Source: CAD feature listing. Evaluate the final solid. Frame: model axes, mm. Coordinates: 2 decimals unless noted, no trailing zeros. Loops run counter-clockwise (first coordinate to the right, second up) from the corner with the lowest first, then second, coordinate; pieces in that order, holes last. Notation, with made-up numbers: (48, 14.25) - (66, 14.25) arc R17 cw to (66, 30.25) - close; hole circle Ø11 at (71.25, 0.25). An arc over 180 degrees is marked (long way). Use CSV: the item, a comma, the result in double quotes. Start each with the question number.
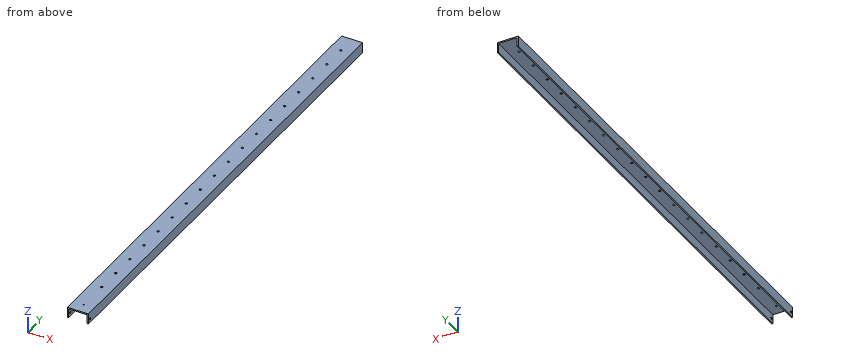
```python
from build123d import *

# Parameters (mm, degrees)
BOSS_EXTRUDE1_DEPTH = 1168.4
IGUS_HOLES_REACH    = 27.4
SKETCH2_R           = 2.667
CUT_EXTRUDE2_REACH  = 5.175
SKETCH3_R           = 1.5875
SKETCH4_R           = 2.667
CUT_EXTRUDE3_DEPTH  = 51.8


with BuildPart() as part:
    # Sketch1 → Boss-Extrude1 (new body)
    with BuildSketch(Plane(origin=(0, 0, 0), x_dir=(1, 0, 0), z_dir=(0, 1, 0))):
        Polygon((3.175, 3.175), (3.175, 25.4), (0, 25.4), (0, 0), (50.8, 0), (50.8, 25.4), (47.625, 25.4), (47.625, 3.175), align=None)
    extrude(amount=BOSS_EXTRUDE1_DEPTH)

    # Sketch2 → Igus_Holes (cut, up to next)
    with BuildSketch(Plane.XY, mode=Mode.PRIVATE) as igus_holes_sk1:
        with Locations((25.4, 101.6)):
            Circle(SKETCH2_R)
    igus_holes_tool1 = extrude(igus_holes_sk1.sketch, amount=-IGUS_HOLES_REACH, mode=Mode.PRIVATE) & part.part
    add(igus_holes_tool1.solids().sort_by_distance((25.4, 101.6, 0))[0], mode=Mode.SUBTRACT)
    # Sketch2 → Igus_Holes (cut, up to next)
    with BuildSketch(Plane.XY, mode=Mode.PRIVATE) as igus_holes_sk2:
        with Locations((25.4, 161.544)):
            Circle(SKETCH2_R)
    igus_holes_tool2 = extrude(igus_holes_sk2.sketch, amount=-IGUS_HOLES_REACH, mode=Mode.PRIVATE) & part.part
    add(igus_holes_tool2.solids().sort_by_distance((25.4, 161.544, 0))[0], mode=Mode.SUBTRACT)
    # Sketch2 → Igus_Holes (cut, up to next)
    with BuildSketch(Plane.XY, mode=Mode.PRIVATE) as igus_holes_sk3:
        with Locations((25.4, 221.488)):
            Circle(SKETCH2_R)
    igus_holes_tool3 = extrude(igus_holes_sk3.sketch, amount=-IGUS_HOLES_REACH, mode=Mode.PRIVATE) & part.part
    add(igus_holes_tool3.solids().sort_by_distance((25.4, 221.488, 0))[0], mode=Mode.SUBTRACT)
    # Sketch2 → Igus_Holes (cut, up to next)
    with BuildSketch(Plane.XY, mode=Mode.PRIVATE) as igus_holes_sk4:
        with Locations((25.4, 281.432)):
            Circle(SKETCH2_R)
    igus_holes_tool4 = extrude(igus_holes_sk4.sketch, amount=-IGUS_HOLES_REACH, mode=Mode.PRIVATE) & part.part
    add(igus_holes_tool4.solids().sort_by_distance((25.4, 281.432, 0))[0], mode=Mode.SUBTRACT)
    # Sketch2 → Igus_Holes (cut, up to next)
    with BuildSketch(Plane.XY, mode=Mode.PRIVATE) as igus_holes_sk5:
        with Locations((25.4, 341.376)):
            Circle(SKETCH2_R)
    igus_holes_tool5 = extrude(igus_holes_sk5.sketch, amount=-IGUS_HOLES_REACH, mode=Mode.PRIVATE) & part.part
    add(igus_holes_tool5.solids().sort_by_distance((25.4, 341.376, 0))[0], mode=Mode.SUBTRACT)
    # Sketch2 → Igus_Holes (cut, up to next)
    with BuildSketch(Plane.XY, mode=Mode.PRIVATE) as igus_holes_sk6:
        with Locations((25.4, 401.32)):
            Circle(SKETCH2_R)
    igus_holes_tool6 = extrude(igus_holes_sk6.sketch, amount=-IGUS_HOLES_REACH, mode=Mode.PRIVATE) & part.part
    add(igus_holes_tool6.solids().sort_by_distance((25.4, 401.32, 0))[0], mode=Mode.SUBTRACT)
    # Sketch2 → Igus_Holes (cut, up to next)
    with BuildSketch(Plane.XY, mode=Mode.PRIVATE) as igus_holes_sk7:
        with Locations((25.4, 461.264)):
            Circle(SKETCH2_R)
    igus_holes_tool7 = extrude(igus_holes_sk7.sketch, amount=-IGUS_HOLES_REACH, mode=Mode.PRIVATE) & part.part
    add(igus_holes_tool7.solids().sort_by_distance((25.4, 461.264, 0))[0], mode=Mode.SUBTRACT)
    # Sketch2 → Igus_Holes (cut, up to next)
    with BuildSketch(Plane.XY, mode=Mode.PRIVATE) as igus_holes_sk8:
        with Locations((25.4, 521.208)):
            Circle(SKETCH2_R)
    igus_holes_tool8 = extrude(igus_holes_sk8.sketch, amount=-IGUS_HOLES_REACH, mode=Mode.PRIVATE) & part.part
    add(igus_holes_tool8.solids().sort_by_distance((25.4, 521.208, 0))[0], mode=Mode.SUBTRACT)
    # Sketch2 → Igus_Holes (cut, up to next)
    with BuildSketch(Plane.XY, mode=Mode.PRIVATE) as igus_holes_sk9:
        with Locations((25.4, 581.152)):
            Circle(SKETCH2_R)
    igus_holes_tool9 = extrude(igus_holes_sk9.sketch, amount=-IGUS_HOLES_REACH, mode=Mode.PRIVATE) & part.part
    add(igus_holes_tool9.solids().sort_by_distance((25.4, 581.152, 0))[0], mode=Mode.SUBTRACT)
    # Sketch2 → Igus_Holes (cut, up to next)
    with BuildSketch(Plane.XY, mode=Mode.PRIVATE) as igus_holes_sk10:
        with Locations((25.4, 641.096)):
            Circle(SKETCH2_R)
    igus_holes_tool10 = extrude(igus_holes_sk10.sketch, amount=-IGUS_HOLES_REACH, mode=Mode.PRIVATE) & part.part
    add(igus_holes_tool10.solids().sort_by_distance((25.4, 641.096, 0))[0], mode=Mode.SUBTRACT)
    # Sketch2 → Igus_Holes (cut, up to next)
    with BuildSketch(Plane.XY, mode=Mode.PRIVATE) as igus_holes_sk11:
        with Locations((25.4, 701.04)):
            Circle(SKETCH2_R)
    igus_holes_tool11 = extrude(igus_holes_sk11.sketch, amount=-IGUS_HOLES_REACH, mode=Mode.PRIVATE) & part.part
    add(igus_holes_tool11.solids().sort_by_distance((25.4, 701.04, 0))[0], mode=Mode.SUBTRACT)
    # Sketch2 → Igus_Holes (cut, up to next)
    with BuildSketch(Plane.XY, mode=Mode.PRIVATE) as igus_holes_sk12:
        with Locations((25.4, 760.984)):
            Circle(SKETCH2_R)
    igus_holes_tool12 = extrude(igus_holes_sk12.sketch, amount=-IGUS_HOLES_REACH, mode=Mode.PRIVATE) & part.part
    add(igus_holes_tool12.solids().sort_by_distance((25.4, 760.984, 0))[0], mode=Mode.SUBTRACT)
    # Sketch2 → Igus_Holes (cut, up to next)
    with BuildSketch(Plane.XY, mode=Mode.PRIVATE) as igus_holes_sk13:
        with Locations((25.4, 820.928)):
            Circle(SKETCH2_R)
    igus_holes_tool13 = extrude(igus_holes_sk13.sketch, amount=-IGUS_HOLES_REACH, mode=Mode.PRIVATE) & part.part
    add(igus_holes_tool13.solids().sort_by_distance((25.4, 820.928, 0))[0], mode=Mode.SUBTRACT)
    # Sketch2 → Igus_Holes (cut, up to next)
    with BuildSketch(Plane.XY, mode=Mode.PRIVATE) as igus_holes_sk14:
        with Locations((25.4, 880.872)):
            Circle(SKETCH2_R)
    igus_holes_tool14 = extrude(igus_holes_sk14.sketch, amount=-IGUS_HOLES_REACH, mode=Mode.PRIVATE) & part.part
    add(igus_holes_tool14.solids().sort_by_distance((25.4, 880.872, 0))[0], mode=Mode.SUBTRACT)
    # Sketch2 → Igus_Holes (cut, up to next)
    with BuildSketch(Plane.XY, mode=Mode.PRIVATE) as igus_holes_sk15:
        with Locations((25.4, 940.816)):
            Circle(SKETCH2_R)
    igus_holes_tool15 = extrude(igus_holes_sk15.sketch, amount=-IGUS_HOLES_REACH, mode=Mode.PRIVATE) & part.part
    add(igus_holes_tool15.solids().sort_by_distance((25.4, 940.816, 0))[0], mode=Mode.SUBTRACT)
    # Sketch2 → Igus_Holes (cut, up to next)
    with BuildSketch(Plane.XY, mode=Mode.PRIVATE) as igus_holes_sk16:
        with Locations((25.4, 1000.76)):
            Circle(SKETCH2_R)
    igus_holes_tool16 = extrude(igus_holes_sk16.sketch, amount=-IGUS_HOLES_REACH, mode=Mode.PRIVATE) & part.part
    add(igus_holes_tool16.solids().sort_by_distance((25.4, 1000.76, 0))[0], mode=Mode.SUBTRACT)
    # Sketch2 → Igus_Holes (cut, up to next)
    with BuildSketch(Plane.XY, mode=Mode.PRIVATE) as igus_holes_sk17:
        with Locations((25.4, 1060.704)):
            Circle(SKETCH2_R)
    igus_holes_tool17 = extrude(igus_holes_sk17.sketch, amount=-IGUS_HOLES_REACH, mode=Mode.PRIVATE) & part.part
    add(igus_holes_tool17.solids().sort_by_distance((25.4, 1060.704, 0))[0], mode=Mode.SUBTRACT)
    # Sketch2 → Igus_Holes (cut, up to next)
    with BuildSketch(Plane.XY, mode=Mode.PRIVATE) as igus_holes_sk18:
        with Locations((25.4, 1120.648)):
            Circle(SKETCH2_R)
    igus_holes_tool18 = extrude(igus_holes_sk18.sketch, amount=-IGUS_HOLES_REACH, mode=Mode.PRIVATE) & part.part
    add(igus_holes_tool18.solids().sort_by_distance((25.4, 1120.648, 0))[0], mode=Mode.SUBTRACT)

    # Sketch3 → Cut-Extrude2 (cut, up to next)
    with BuildSketch(Plane(origin=(0, 0, -3.175), x_dir=(-1, 0, 0), z_dir=(0, 0, -1)), mode=Mode.PRIVATE) as cut_extrude2_sk1:
        with Locations((-25.4, 25.4)):
            Circle(SKETCH3_R)
    cut_extrude2_tool1 = extrude(cut_extrude2_sk1.sketch, amount=-CUT_EXTRUDE2_REACH, mode=Mode.PRIVATE) & part.part
    add(cut_extrude2_tool1.solids().sort_by_distance((25.4, 25.4, -3.175))[0], mode=Mode.SUBTRACT)

    # Sketch4 → Cut-Extrude3 (cut, through all)
    with BuildSketch(Plane.ZY):
        with Locations((-15.875, 6.35)):
            Circle(SKETCH4_R)
    extrude(amount=-CUT_EXTRUDE3_DEPTH, mode=Mode.SUBTRACT)


solid = part.part
```
(1) Pin query (flat end, axial travel): pin 1 Ø7 at (x, y) = (25.4, 341.376) entering from -Z (3 decimals). Return the tip coordinate at first contact, or that it passes through.
(2) Section B-B on y = 131. Output: boundary loops of the cut face in (x, z) (3 decimals), plus the area to 3 significant figures.
(3) Section A-A on z = -8. Output: boundary loops of the cut face in (x, y) (3 decimals), plus the area to 3 significant figures.
(4) Ray query, line 1 (X direction, y = 491.5, z = -10.5) (3 decimals); line 2 (Z direction, x = 34.5, y = 450) (3 decimals). Return the intervals inside material, ascending. Write a range as [from, to].
Solution:
1,pin 1,"stops at z = -3.175"
2,outline,"(0, -25.4) - (3.175, -25.4) - (3.175, -3.175) - (47.625, -3.175) - (47.625, -25.4) - (50.8, -25.4) - (50.8, 0) - (0, 0) - close"
2,area,"302 mm²"
3,outline,"(0, 0) - (3.175, 0) - (3.175, 1168.4) - (0, 1168.4) - close; (47.625, 0) - (50.8, 0) - (50.8, 1168.4) - (47.625, 1168.4) - close"
3,area,"7,420 mm²"
4,line 1,"x = [0, 3.175], [47.625, 50.8]"
4,line 2,"z = [-3.175, 0]"
